The listing builds one solid part. Answer for the finished solid, in the listing's coordinates (mm). Face numbers are marked on the shaded views. A direction names the side the tool comes from. Round coordinates to 2 decimals unless told otherwise and drop trailing zeros. Order: outer loops, then holes, each group sorted by start corner. A loop starts at its lowest first (then second) coordinate and runs counter-clockwise, first axis right, second up. Notation, with made-up numbers: M 46.25,48.5 L 62.25,48.5 A19 cw 62.25,66.5 Z; hole C 68.25,-27.75 d9. An arc over 180 degrees is marked long. Write item = value, one per line. Start each with the question number.
(1) A cutting plane is placed at B-B, the plane x = -2. Determine the outline of the cut face in (y, z).
(2) Each of these flat-tipped pins is pushed along its axis until it touches: pin 1 (1.1 mm diameter, centred on y = 2, z = 0.5, fed in from +X); pin 2 (0.8 mm diameter, centred on x = 2.5, z = 0.5, fed in from +Y); pin 3 (3 mm diameter, centred on x = 1, z = 0, fed in from +Y). Where does it stop, or does it pass through?
(3) Which of the six approach directions +Z, -Z, +X, -X, +Y, -Y give full straight-line access (tool end or side, diameter ignored) to the marked faces 5, 6, 7, 8 and 9?
(4) Straight lines are drawn through the part: probe 1 along Z at (x, y) = (1.75, 0.55); probe 2 along Z at (x, y) = (-0.5, 4.3); probe 3 along X at (y, z) = (0.4, -1.75). For each, find the intervals that lie inside material, in ascending order. Write a range as from..to.
(5) A cutting plane is placed at A-A, the plane y = 1.05. Determine the outline of the cut face in (x, z).
(6) For a pull along X with two mould halves and no side action, classify the marked faces 1, 2, 3 and 4 as released by +X, released by -X, zero draft, split by the parting line, or undercut.
(7) A cutting plane is placed at D-D, the plane x = 2.75. Determine the outline of the cut face in (y, z).
(8) A cutting plane is placed at C-C, the plane z = 1. Determine the outline of the cut face in (x, y) (3 decimals), and give its area (3 significant figures).
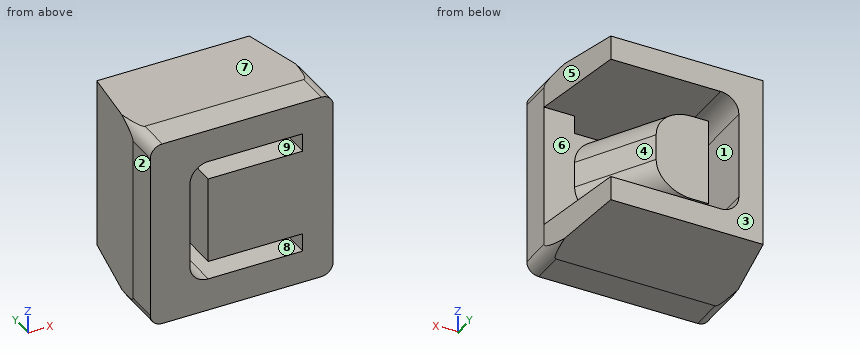
from build123d import *

# Parameters (mm, degrees)
EXTRUDE1_DEPTH      = 3.937
DRAFT1_START        = -3.81
DRAFT1_DEPTH        = 7.62
SKETCH3_W           = 5.969
SKETCH3_H           = 5.144225416
CUT_EXTRUDE1_DEPTH  = 16.999459798
CUT_EXTRUDE2_DEPTH  = 16.999459798
SKETCH5_W           = 3.937
SKETCH5_H           = 3.620225416
EXTRUDE2_DEPTH      = 3.048
DRAFT2_ANGLE        = 30
FILLET1_R           = 1.27
FILLET2_R           = 0.762
SKETCH6_W           = 3.937
SKETCH6_H           = 3.620225416
EXTRUDE3_DEPTH      = 1.3462
CUT_EXTRUDE3_DEPTH  = 16.999459798
SKETCH12_W          = 4.3942
SKETCH12_H          = 1.3462
BOSS_EXTRUDE1_DEPTH = 70
CUT_EXTRUDE8_DEPTH  = 1.524
LPATTERN1_START     = -1.524
LPATTERN1_DEPTH     = 3.048
CUT_EXTRUDE9_DEPTH  = 86.170550743
FILLET3_R           = 1
CUT_EXTRUDE10_DEPTH = 85.172743295
FILLET4_R           = 0.5
CUT_EXTRUDE11_START = -1.3462
CUT_EXTRUDE11_DEPTH = 1.3462


# Read off the part's stored shape, not the designer's step: Draft1, LPattern1, Cut-Extrude11
with BuildPart() as part:
    # Sketch1 → Extrude1 (new, symmetric)
    with BuildSketch(Plane.XY):
        Polygon((3.81, 1.3462), (3.175, 5.334), (-3.175, 5.334), (-3.81, 1.3462), (-3.81, 0), (14.986, 0), (14.986, 1.3462), align=None)
    extrude(amount=EXTRUDE1_DEPTH, both=True)

    # Draft1 outline → Draft1 (cut)
    with BuildSketch(Plane.YZ.offset(DRAFT1_START)):
        Polygon((1.3462, 3.937), (5.334, 3.588112708), (5.334, 3.937), align=None)
        Polygon((5.334, -3.588112708), (1.3462, -3.937), (5.334, -3.937), align=None)
    extrude(amount=DRAFT1_DEPTH, mode=Mode.SUBTRACT)

    # Sketch3 → Cut-Extrude1 (cut, through all)
    with BuildSketch(Plane(origin=(0, 1.3462, 0), x_dir=(-1, 0, 0), z_dir=(0, 1, 0))):
        with Locations((-0.8255, 0)):
            Rectangle(SKETCH3_W, SKETCH3_H)
    extrude(amount=CUT_EXTRUDE1_DEPTH, mode=Mode.SUBTRACT)

    # Sketch4 → Cut-Extrude2 (cut, through all)
    with BuildSketch(Plane(origin=(0, 1.3462, 0), x_dir=(-1, 0, 0), z_dir=(0, 1, 0))):
        Polygon((2.159, 2.572112708), (-2.54, 2.572112708), (-2.54, 1.810112708), (1.397, 1.810112708), (1.397, -1.810112708), (-2.54, -1.810112708), (-2.54, -2.572112708), (2.159, -2.572112708), align=None)
    extrude(amount=-CUT_EXTRUDE2_DEPTH, mode=Mode.SUBTRACT)

    # Sketch5 → Extrude2 (add)
    with BuildSketch(Plane(origin=(0, 1.3462, 0), x_dir=(-1, 0, 0), z_dir=(0, 1, 0))):
        with Locations((-0.5715, 0)):
            Rectangle(SKETCH5_W, SKETCH5_H)
    extrude(amount=EXTRUDE2_DEPTH)

    # Draft2
    draft2_faces = [part.faces().sort_by_distance(p)[0] for p in [
        (2.54, 2.8702, 0),
    ]]
    draft(draft2_faces, Plane(origin=(14.986, 1.3462, 3.937), x_dir=(1, 0, 0), z_dir=(0, 1, 0)), DRAFT2_ANGLE)

    # Fillet1
    # the kernel refuses this fillet: 1.27 mm, written as the material it takes off along each edge
    with BuildSketch(Plane(origin=(4.1275, -1.403430657, 1.810112708), x_dir=(-0.866025403784438, -0.500000000000001, 0), z_dir=(-0.500000000000001, 0.866025403784438, 0))) as fillet1_piece_1_section:
        with BuildLine():
            CenterArc((FILLET1_R, -FILLET1_R), FILLET1_R, 90, 90)
            Line((0, -FILLET1_R), (0, 0))
            Line((0, 0), (FILLET1_R, 0))
        make_face()
    fillet1_piece_1 = extrude(amount=9.869527241, mode=Mode.PRIVATE)
    fillet1_piece_1 = split(fillet1_piece_1, bisect_by=Plane(origin=(2.54, 0.912532514, 1.637821639), z_dir=(-1, 0, 0)), keep=Keep.TOP, mode=Mode.PRIVATE)
    add(fillet1_piece_1, mode=Mode.SUBTRACT)
    with BuildSketch(Plane(origin=(4.1275, -1.403430657, -1.810112708), x_dir=(-0.8660254037844382, -0.500000000000001, 0), z_dir=(-0.500000000000001, 0.866025403784438, 0))) as fillet1_piece_2_section:
        with BuildLine():
            CenterArc((FILLET1_R, FILLET1_R), FILLET1_R, 180, 90)
            Line((0, FILLET1_R), (0, 0))
            Line((0, 0), (FILLET1_R, 0))
        make_face()
    fillet1_piece_2 = extrude(amount=9.869527241, mode=Mode.PRIVATE)
    fillet1_piece_2 = split(fillet1_piece_2, bisect_by=Plane(origin=(2.54, 0.912532514, -1.637821639), z_dir=(-1, 0, 0)), keep=Keep.TOP, mode=Mode.PRIVATE)
    add(fillet1_piece_2, mode=Mode.SUBTRACT)

    # Fillet2
    fillet2_edges = [part.edges().sort_by_distance(p)[0] for p in [
        (-2.159, 2.667, 2.572112708),
        (-2.159, 2.667, -2.572112708),
    ]]
    fillet(fillet2_edges, radius=FILLET2_R)

    # Sketch6 → Extrude3 (add)
    with BuildSketch(Plane.XZ):
        with Locations((0.5715, 0)):
            Rectangle(SKETCH6_W, SKETCH6_H)
    extrude(amount=-EXTRUDE3_DEPTH)

    # Sketch7 → Cut-Extrude3 (cut, through all)
    with BuildSketch(Plane(origin=(0, 1.3462, 0), x_dir=(-1, 0, 0), z_dir=(0, 1, 0))):
        Polygon((-14.986, 3.937), (-3.81, 3.937), (-10.668, 2.1971), (-14.986, 2.1971), align=None)
        Polygon((-14.986, -3.937), (-3.81, -3.937), (-10.668, -2.1971), (-14.986, -2.1971), align=None)
    extrude(amount=-CUT_EXTRUDE3_DEPTH, mode=Mode.SUBTRACT)

    # Sketch12 → Boss-Extrude1 (add)
    with BuildSketch(Plane(origin=(14.986, 0, 0), x_dir=(0, 0, -1), z_dir=(1, 0, 0))):
        with Locations((0, 0.6731)):
            Rectangle(SKETCH12_W, SKETCH12_H)
    extrude(amount=BOSS_EXTRUDE1_DEPTH)

    # Sketch11 → Cut-Extrude8 (cut, symmetric)
    with BuildSketch(Plane.XY):
        Polygon((10.668, 1.3462), (10.668, 1.0922), (11.684, 1.3462), (11.684, 1.637608524), (10.668, 1.637608524), align=None)
    extrude(amount=CUT_EXTRUDE8_DEPTH, both=True, mode=Mode.SUBTRACT)

    # LPattern1 outline → LPattern1 (cut)
    with BuildSketch(Plane.XY.offset(LPATTERN1_START)):
        Polygon((14.184, 1.3462), (13.168, 1.3462), (13.168, 1.0922), align=None)
        Polygon((79.184, 1.3462), (78.168, 1.3462), (78.168, 1.0922), align=None)
        Polygon((76.684, 1.3462), (75.668, 1.3462), (75.668, 1.0922), align=None)
        Polygon((74.184, 1.3462), (73.168, 1.3462), (73.168, 1.0922), align=None)
        Polygon((71.684, 1.3462), (70.668, 1.3462), (70.668, 1.0922), align=None)
        Polygon((69.184, 1.3462), (68.168, 1.3462), (68.168, 1.0922), align=None)
        Polygon((66.684, 1.3462), (65.668, 1.3462), (65.668, 1.0922), align=None)
        Polygon((64.184, 1.3462), (63.168, 1.3462), (63.168, 1.0922), align=None)
        Polygon((61.684, 1.3462), (60.668, 1.3462), (60.668, 1.0922), align=None)
        Polygon((59.184, 1.3462), (58.168, 1.3462), (58.168, 1.0922), align=None)
        Polygon((56.684, 1.3462), (55.668, 1.3462), (55.668, 1.0922), align=None)
        Polygon((54.184, 1.3462), (53.168, 1.3462), (53.168, 1.0922), align=None)
        Polygon((51.684, 1.3462), (50.668, 1.3462), (50.668, 1.0922), align=None)
        Polygon((49.184, 1.3462), (48.168, 1.3462), (48.168, 1.0922), align=None)
        Polygon((46.684, 1.3462), (45.668, 1.3462), (45.668, 1.0922), align=None)
        Polygon((44.184, 1.3462), (43.168, 1.3462), (43.168, 1.0922), align=None)
        Polygon((41.684, 1.3462), (40.668, 1.3462), (40.668, 1.0922), align=None)
        Polygon((39.184, 1.3462), (38.168, 1.3462), (38.168, 1.0922), align=None)
        Polygon((36.684, 1.3462), (35.668, 1.3462), (35.668, 1.0922), align=None)
        Polygon((34.184, 1.3462), (33.168, 1.3462), (33.168, 1.0922), align=None)
        Polygon((31.684, 1.3462), (30.668, 1.3462), (30.668, 1.0922), align=None)
        Polygon((29.184, 1.3462), (28.168, 1.3462), (28.168, 1.0922), align=None)
        Polygon((26.684, 1.3462), (25.668, 1.3462), (25.668, 1.0922), align=None)
        Polygon((24.184, 1.3462), (23.168, 1.3462), (23.168, 1.0922), align=None)
        Polygon((21.684, 1.3462), (20.668, 1.3462), (20.668, 1.0922), align=None)
        Polygon((19.184, 1.3462), (18.168, 1.3462), (18.168, 1.0922), align=None)
        Polygon((16.684, 1.3462), (15.668, 1.3462), (15.668, 1.0922), align=None)
    extrude(amount=LPATTERN1_DEPTH, mode=Mode.SUBTRACT)

    # Sketch13 → Cut-Extrude9 (cut, through all)
    with BuildSketch(Plane(origin=(0, 1.3462, 0), x_dir=(1, 0, 0), z_dir=(0, 1, 0))):
        Polygon((84.986, -2.1971), (84.986, 0), (81.180511171, -2.1971), align=None)
        Polygon((81.180511171, 2.1971), (84.986, 0), (84.986, 2.1971), align=None)
    extrude(amount=-CUT_EXTRUDE9_DEPTH, mode=Mode.SUBTRACT)

    # Fillet3
    fillet3_edges = [part.edges().sort_by_distance(p)[0] for p in [
        (84.986, 0.6731, 0),
    ]]
    fillet(fillet3_edges, radius=FILLET3_R)

    # Sketch14 → Cut-Extrude10 (cut, through all)
    with BuildSketch(Plane(origin=(0, 1.3462, 0), x_dir=(1, 0, 0), z_dir=(0, 1, 0))):
        Polygon((10.668, 2.1971), (3.81, 2.1971), (3.81, 3.937), align=None)
    cut_extrude10 = extrude(amount=-CUT_EXTRUDE10_DEPTH, mode=Mode.SUBTRACT)

    # Mirror1: Cut-Extrude10 across plane
    add(cut_extrude10.mirror(Plane.XY), mode=Mode.SUBTRACT)

    # Fillet4
    # the kernel refuses this fillet: 0.5 mm, written as the material it adds along each edge
    with BuildSketch(Plane(origin=(3.81, 1.3462, -2.1971), x_dir=(1, 0, 0), z_dir=(0, -1, 0)), Plane(origin=(3.81, 1.3462, 2.1971), x_dir=(0, 0, 1), z_dir=(0, -1, 0))) as fillet4_piece_1:
        with BuildLine():
            CenterArc((FILLET4_R, -FILLET4_R), FILLET4_R, 90, 90)
            Line((0, -FILLET4_R), (0, 0))
            Line((0, 0), (FILLET4_R, 0))
        make_face()
    extrude(amount=1.3462)
    # the kernel refuses this fillet: 0.5 mm, written as the material it takes off along each edge
    with BuildSketch(Plane(origin=(3.81, 2.5962, 3.937), x_dir=(0, 0, -1), z_dir=(0, -1, 0)), Plane(origin=(-3.81, 2.5962, 3.937), x_dir=(1, 0, 0), z_dir=(0, -1, 0)), Plane(origin=(3.81, 2.5962, -3.937), x_dir=(-1, 0, 0), z_dir=(0, -1, 0)), Plane(origin=(-3.81, 2.5962, -3.937), x_dir=(0, 0, 1), z_dir=(0, -1, 0))) as fillet4_2_piece_1:
        with BuildLine():
            CenterArc((FILLET4_R, -FILLET4_R), FILLET4_R, 90, 90)
            Line((0, -FILLET4_R), (0, 0))
            Line((0, 0), (FILLET4_R, 0))
        make_face()
    extrude(amount=3.8462, mode=Mode.SUBTRACT)

    # Cut-Extrude11 outline → Cut-Extrude11 (cut)
    with BuildSketch(Plane(origin=(0, 1.3462, 0), x_dir=(1, 0, 0), z_dir=(0, 1, 0)).offset(CUT_EXTRUDE11_START)):
        with BuildLine():
            ThreePointArc((4.31, 2.1971), (3.956446609, 2.343546609), (3.81, 2.6971))
            Line((3.81, 2.6971), (3.81, -2.6971))
            ThreePointArc((3.81, -2.6971), (3.956446609, -2.343546609), (4.31, -2.1971))
            Line((4.31, -2.1971), (81.180511171, -2.1971))
            Line((81.180511171, -2.1971), (83.486, -0.866025404))
            ThreePointArc((83.486, -0.866025404), (83.986, 0), (83.486, 0.866025404))
            Line((83.486, 0.866025404), (81.180511171, 2.1971))
            Line((81.180511171, 2.1971), (4.31, 2.1971))
        make_face()
    extrude(amount=CUT_EXTRUDE11_DEPTH, mode=Mode.SUBTRACT)


solid = part.part
Reported:
q1.outline = M 0,-3.94 L 1.35,-3.94 L 5.33,-3.59 L 5.33,-2.28 L 0,-2.28 Z; M 0,2.28 L 5.33,2.28 L 5.33,3.59 L 1.35,3.94 L 0,3.94 Z
q2.pin_1 = 2.48
q2.pin_2 = 2.11
q2.pin_3 = 4.39
q3.face_5 = +Z, -Z, +X, +Y
q3.face_6 = +X, +Y
q3.face_7 = +Z, +X, -X, +Y
q3.face_8 = +Y
q3.face_9 = +Y, -Y
q4.probe_1 = -3.94..-2.57, -1.81..1.81, 2.57..3.94
q4.probe_2 = -3.68..-2.57, -1.8..1.8, 2.57..3.68
q4.probe_3 = -3.81..-2.16, -1.4..3.81
q5.outline = M -3.81,-3.44 A0.5 ccw -3.31,-3.94 L 3.31,-3.94 A0.5 ccw 3.81,-3.44 L 3.81,3.44 A0.5 ccw 3.31,3.94 L -3.31,3.94 A0.5 ccw -3.81,3.44 Z; hole M -2.16,-1.81 A0.76 ccw -1.4,-2.57 L 2.54,-2.57 L 2.54,-1.81 L -1.4,-1.81 L -1.4,1.81 L 2.54,1.81 L 2.54,2.57 L -1.4,2.57 A0.76 ccw -2.16,1.81 Z
q6.face_1 = undercut
q6.face_2 = released by -X
q6.face_3 = zero draft
q6.face_4 = released by +X
q7.outline = M 0,-3.94 L 1.35,-3.94 L 5.33,-3.59 L 5.33,-2.57 L 1.35,-2.57 L 1.35,2.57 L 5.33,2.57 L 5.33,3.59 L 1.35,3.94 L 0,3.94 Z
q8.outline = M -3.81,0 L -2.159,0 L -2.159,5.334 L -3.175,5.334 L -3.81,1.346 Z; M -1.397,0 L 3.81,0 L 3.81,1.346 L 2.44,1.346 L 0.681,4.394 L -1.397,4.394 Z
q8.area = 23.6 mm²
